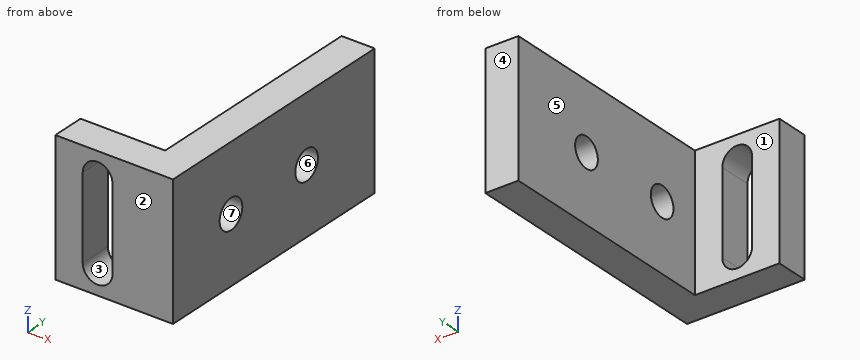
```python
from build123d import *

# Parameters (mm, degrees)
RESSALTO_EXTRUS_O1_DEPTH = 20
CORTE_EXTRUS_O1_DEPTH    = 45.05823873
ESBO_O3_R                = 2.25
CORTE_EXTRUS_O2_DEPTH    = 47.511594253


with BuildPart() as part:
    # Esboço1 → Ressalto-extrusão1 (new body)
    with BuildSketch(Plane.XY):
        Polygon((0, 0), (0, 5), (12.78, 5), (12.78, 40), (17.78, 40), (17.78, 0), align=None)
    extrude(amount=RESSALTO_EXTRUS_O1_DEPTH)

    # Esboço2 → Corte-extrusão1 (cut, through all)
    with BuildSketch(Plane(origin=(0, 5, 0), x_dir=(1, 0, 0), z_dir=(0, 1, 0))):
        with BuildLine():
            Line((8.64, -3.75), (8.64, -16.25))
            ThreePointArc((8.64, -16.25), (6.39, -18.5), (4.14, -16.25))
            Line((4.14, -16.25), (4.14, -3.75))
            ThreePointArc((4.14, -3.75), (6.39, -1.5), (8.64, -3.75))
        make_face()
    extrude(amount=-CORTE_EXTRUS_O1_DEPTH, mode=Mode.SUBTRACT)

    # Esboço3 → Corte-extrusão2 (cut, through all)
    with BuildSketch(Plane.ZY.offset(-12.78)):
        with Locations((10, 26.5)):
            Circle(ESBO_O3_R)
        with Locations((10, 11.5)):
            Circle(ESBO_O3_R)
    extrude(amount=-CORTE_EXTRUS_O2_DEPTH, mode=Mode.SUBTRACT)


solid = part.part
```
Geometry: final body of the model. Coordinates: model frame, mm. Face numbers are marked on the shaded views. A direction names the side the tool comes from. Round coordinates to 2 decimals unless told otherwise and drop trailing zeros. Order: outer loops, then holes, each group sorted by start corner. A loop starts at its lowest first (then second) coordinate and runs counter-clockwise, first axis right, second up. Notation, with made-up numbers: (72, -33) -> (108, -33) arc R38 ccw to (108, 6) -> close; hole circle Ø9 at (26.5, 51). An arc over 180 degrees is marked (long way). Write each question's results on one line, items separated by ' | '.
Q1. Section query A-A (y = 11.5). Output: boundary loops of the cut face in (x, z).
Response values:
outline: (12.78, 0) -> (17.78, 0) -> (17.78, 7.75) -> (12.78, 7.75) -> close; (12.78, 12.25) -> (17.78, 12.25) -> (17.78, 20) -> (12.78, 20) -> close
Q2. Pin query (flat end, axial travel): pin 1 Ø6 at (y, z) = (21.5, 9.5) entering from -X; pin 2 Ø8 at (x, z) = (3, 4.5) entering from +Y. Return the tip coordinate at first contact, or that it passes through.
Response values:
pin 1: x = 12.78 | pin 2: y = 5
Q3. Section query B-B (z = 4.25). Output: boundary loops of the cut face in (x, y).
Response values:
outline: (0, 0) -> (4.14, 0) -> (4.14, 5) -> (0, 5) -> close; (8.64, 0) -> (17.78, 0) -> (17.78, 40) -> (12.78, 40) -> (12.78, 5) -> (8.64, 5) -> close
Q4. Section query C-C (z = 10). Output: boundary loops of the cut face in (x, y), and give its area (3 significant figures).
Response values:
outline: (0, 0) -> (4.14, 0) -> (4.14, 5) -> (0, 5) -> close; (8.64, 0) -> (17.78, 0) -> (17.78, 9.25) -> (12.78, 9.25) -> (12.78, 5) -> (8.64, 5) -> close; (12.78, 13.75) -> (17.78, 13.75) -> (17.78, 24.25) -> (12.78, 24.25) -> close; (12.78, 28.75) -> (17.78, 28.75) -> (17.78, 40) -> (12.78, 40) -> close | area: 196 mm²
Q5. Access query for the marked faces 1, 2 and 3. Directions: +Z, -Z, +X, -X, +Y, -Y. A direction counts if a zero-diameter tool reaches every point of the face in a straight line with its end or side. Return the directions, or none.
Response values:
face 1: +Z, -Z, -X, +Y | face 2: +Z, -Z, +X, -X, -Y | face 3: +Y, -Y
Q6. Ray query, line 1 along Y through (x, z) = (15.65, 10); line 2 along X through (y, z) = (2, 15); line 3 along X through (y, z) = (11, 3.25). Return the intervals inside material, ascending.
Response values:
line 1: 0 to 9.25, 13.75 to 24.25, 28.75 to 40 | line 2: 0 to 4.14, 8.64 to 17.78 | line 3: 12.78 to 17.78
Q7. Section query D-D (x = 5). Output: boundary loops of the cut face in (y, z), and give its area (3 significant figures).
Response values:
outline: (0, 0) -> (5, 0) -> (5, 1.98) -> (0, 1.98) -> close; (0, 18.02) -> (5, 18.02) -> (5, 20) -> (0, 20) -> close | area: 19.8 mm²
Q8. Pull-direction query (Y, two-part tool) for the marked faces 4, 5, 6 and 7; classes: released by +Y, released by -Y, zero draft, split by the parting line, or undercut.
Response values:
face 4: released by +Y | face 5: zero draft | face 6: undercut | face 7: undercut
